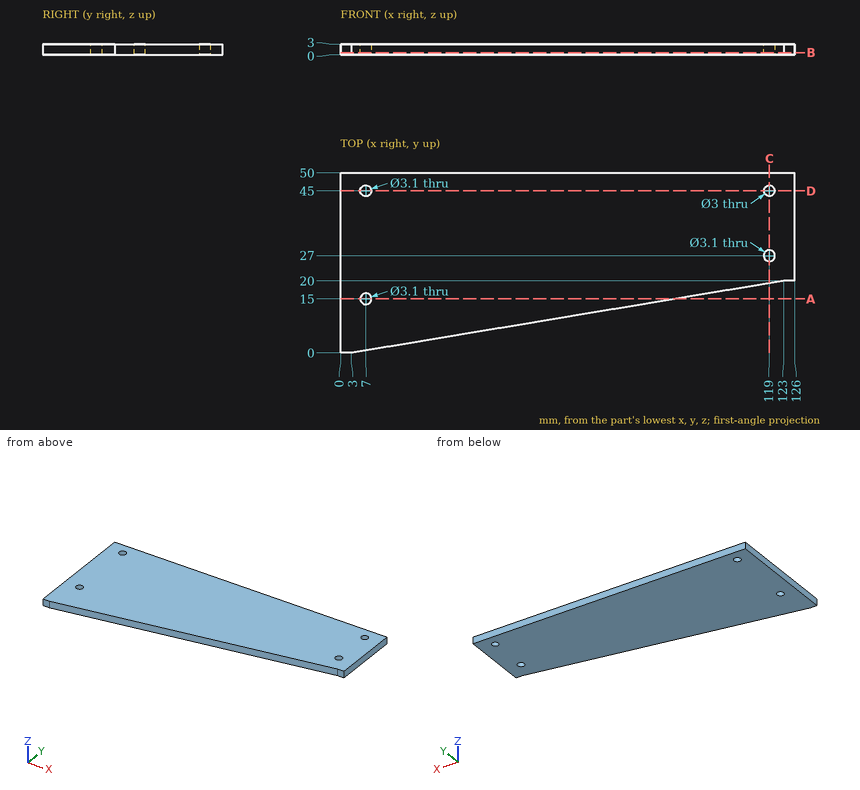
The drawing under review shows one solid part. Ordinate dimensions are in mm from its lowest x, y, z. Coordinates: 2 decimals unless noted, no trailing zeros. Write each loop counter-clockwise with the first axis right and the second up, starting at its lowest first coordinate (ties: lowest second). Pieces come first, ordered by that corner, then holes.
1) Add section C-C (x = 119). Write out the cut boundary in (y, z).
2) Insertion check: pin 1 (4 mm diameter, centred on x = 119, y = 45, fed in from -Z); pin 2 (1.5 mm diameter, centred on x = 98.5, z = 2, fed in from -Y). Each pin has a flat end and moves straight along its axis. Give the tip position at first contact, or say it passes through.
3) Add section B-B (z = 0.6). Write out the cut boundary in (x, y).
4) Add section D-D (y = 45). Write out the cut boundary in (x, z).
5) Add section A-A (y = 15). Write out the cut boundary in (x, z).
6) To check wall thickness, follow L1, parallel to Y at x = 119, z = 1.3; L2, parallel to Y at x = 55, z = 1.35; L3, parallel to Y at x = 114.5, z = 1.65. State the ranges of each line that lie inside material, in increasing order.
Check result:
1. outline: (19.33, 0) - (25.45, 0) - (25.45, 3) - (19.33, 3) - close; (28.55, 0) - (43.5, 0) - (43.5, 3) - (28.55, 3) - close; (46.5, 0) - (50, 0) - (50, 3) - (46.5, 3) - close
2. pin 1: stops at z = 0
2. pin 2: stops at y = 15.79
3. outline: (0, 0) - (3, 0) - (123, 20) - (126, 20) - (126, 50) - (0, 50) - close; hole circle Ø3.1 at (7, 15); hole circle Ø3.1 at (7, 45); hole circle Ø3.1 at (119, 27); hole circle Ø3 at (119, 45)
4. outline: (0, 0) - (5.45, 0) - (5.45, 3) - (0, 3) - close; (8.55, 0) - (117.5, 0) - (117.5, 3) - (8.55, 3) - close; (120.5, 0) - (126, 0) - (126, 3) - (120.5, 3) - close
5. outline: (0, 0) - (5.45, 0) - (5.45, 3) - (0, 3) - close; (8.55, 0) - (93, 0) - (93, 3) - (8.55, 3) - close
6. L1: y = 19.33 to 25.45, 28.55 to 43.5, 46.5 to 50
6. L2: y = 8.67 to 50
6. L3: y = 18.58 to 50
